from build123d import *

# Parameters (mm, degrees)
BOSS_EXTRUDE1_DEPTH = 700
FILLET4_R           = 50
FILLET5_R           = 50
BOSS_EXTRUDE2_DEPTH = 5


with BuildPart() as part:
    # Sketch1 → Boss-Extrude1 (new body)
    with BuildSketch(Plane.XY):
        Polygon((0, 0), (-120, 0), (-500.276363355, 64.455479422), (-80.272969111, 321.336979592), (-80.272969111, 326.336979592), (-506.593051288, 65.087697234), (-512.515194277, 61.458603343), (-505.351292424, 60.244347678), (-120.420740562, -5), (0, -5), align=None)
    extrude(amount=BOSS_EXTRUDE1_DEPTH)

    # Fillet4
    fillet4_edges = [part.edges().sort_by_distance(p)[0] for p in [
        (-500.276363355, 64.455479422, 350),
    ]]
    fillet(fillet4_edges, radius=FILLET4_R)

    # Fillet5
    fillet5_edges = [part.edges().sort_by_distance(p)[0] for p in [
        (-512.515194277, 61.458603343, 350),
    ]]
    fillet(fillet5_edges, radius=FILLET5_R)

    # Sketch2 → Boss-Extrude2 (add)
    with BuildSketch(Plane.XY.offset(700)):
        with BuildLine():
            Line((-120.420740562, -5), (-381.084420098, 39.181558602))
            add(Edge.make_bspline(
                [(-398.853702629, 131.110455006), (-406.706116268, 126.337398714), (-417.396955451, 114.668240543), (-424.220724955, 91.713060572), (-421.112435822, 70.320363039), (-406.882601787, 49.048758298), (-391.360070335, 40.876151559), (-381.084420098, 39.181558602)],
                knots=[0, 0, 0, 0, 0.228119285, 0.378356265, 0.583675291, 0.742972739, 1, 1, 1, 1], degree=3))
            Line((-398.853702629, 131.110455006), (-80.272969111, 326.336979592))
            Line((-80.272969111, 326.336979592), (-80.272969111, 0))
            Line((-80.272969111, 0), (-80.272969111, -5))
            Line((-80.272969111, -5), (-120.420740562, -5))
        make_face()
    extrude(amount=-BOSS_EXTRUDE2_DEPTH)

    # Mirror2: part across plane


with BuildPart() as part_1:
    add(part.part)
    add(part.part.mirror(Plane.XY.offset(350)))


solid = part_1.part
Here's how the part is built. I have some questions about the finished solid (model axes, mm). A direction names the side the tool comes from. Give positions to 0.01 mm unless a question says otherwise; leave off trailing zeros. Loops run counter-clockwise (first coordinate to the right, second up) from the corner with the lowest first, then second, coordinate; pieces in that order, holes last. Notation, with made-up numbers: (28, 38) -> (81, 38) arc R32 ccw to (81, 65) -> close; hole circle Ø10 at (56, 39.5). An arc over 180 degrees is marked (long way). Answer as a JSON object with one key per item and string values. Group by question number.
Item 1: Imagine slicing it at B-B on y = 255. Write out the boundary of the cut face in (x, z).
Item 2: Imagine slicing it at C-C on x = -189. Write out the boundary of the cut face in (y, z), then the cut area to 3 significant figures.
Item 3: On a 3-axis mill with a long thin cutter (end or side, diameter ignored), from which of +Z, -Z, +X, -X, +Y, -Y can I reach the whole of each face in a straight line? I mean faces 1 (the flat face through (-61, -5, 345)), 2 (the flat face through (-235.48, 226.41, 345.17)). Say none if no direction works.
Item 4: Imagine slicing it at A-A on x = -310. Write out the boundary of the cut face in (y, z).
Item 5: Will these pins go through, and if not, where does the flat tip stop? pin 1 (12 mm diameter, centred on y = 39.5, z = 463.5, fed in from -X); pin 2 (8 mm diameter, centred on y = 133, z = 318.5, fed in from +X); pin 3 (4 mm diameter, centred on x = -237, z = 439, fed in from -Y).
Item 6: Imagine slicing it at D-D on x = -39.5. Write out the boundary of the cut face in (y, z), then the cut area to 3 significant figures.
Item 7: I need wall thicknesses on L1, parallel to Z at x = -211, y = 161.5; L2, parallel to Y at x = -394, z = 551; L3, parallel to Y at x = -36, z = 212.5. Which ranges of each line are inside material? Lowest first, please.
Item 8: Thinking about a two-plate mould opening in Z: for faces 3 (the flat face through (-252.58, 17.4, 345.1)), 4 (the cylindrical face through (-409.245, 81.146, 354.83)), 5 (the flat face through (-214, 126, 700)), 6 (the flat face through (-214, 126, 0)), which applies, pulls with the +Z half, pulls with the -Z half, needs draft (parallel to the pull), parting line crosses it, or undercut?
Answer list:
{
 "1": {"outline": "(-196.68, 0) -> (-80.27, 0) -> (-80.27, 5) -> (-188.73, 5) -> (-188.73, 695) -> (-80.27, 695) -> (-80.27, 700) -> (-196.68, 700) -> close"},
 "2": {"outline": "(6.62, 0) -> (259.71, 0) -> (259.71, 700) -> (6.62, 700) -> close; hole (11.7, 5) -> (254.84, 5) -> (254.84, 695) -> (11.7, 695) -> close", "area": "9,390 mm2"},
 "3": {"face 1": "+Z, -Z, +X, -X, -Y", "face 2": "+X"},
 "4": {"outline": "(27.13, 0) -> (185.56, 0) -> (185.56, 700) -> (27.13, 700) -> close; hole (32.2, 5) -> (180.83, 5) -> (180.83, 695) -> (32.2, 695) -> close"},
 "5": {"pin 1": "stops at x = -398.28", "pin 2": "stops at x = -381.67", "pin 3": "stops at y = 14.42"},
 "6": {"outline": "(-5, 0) -> (0, 0) -> (0, 700) -> (-5, 700) -> close", "area": "3,500 mm2"},
 "7": {"L1": "z = 0 to 5, 695 to 700", "L2": "y = 43.23 to 54.49, 128.4 to 134.08", "L3": "y = -5 to 0"},
 "8": {"face 3": "needs draft", "face 4": "undercut", "face 5": "pulls with the +Z half", "face 6": "pulls with the -Z half"}
}
